Work out the finished part from the listing and answer in its coordinate system (mm). Face numbers are marked on the shaded views. A direction names the side the tool comes from. Give positions to 0.01 mm unless a question says otherwise; leave off trailing zeros. Write each loop counter-clockwise with the first axis right and the second up, starting at its lowest first coordinate (ties: lowest second). Pieces come first, ordered by that corner, then holes.
1) Find section D-D (z = -12.5). Determine the outline of the cut face in (x, y) (3 decimals).
2) Determine the mould class of the marked faces 1, 2 and 3 for opening direction Y: pulls with the +Y half, pulls with the -Y half, needs draft (parallel to the pull), parting line crosses it, or undercut.
3) Find section A-A (y = -3). Determine the outline of the cut face in (x, z).
4) Straight lines are drawn through the part: probe 1 along Z at (x, y) = (-17.5, 8.5); probe 2 along Z at (x, y) = (19.5, 18); probe 3 along X at (y, z) = (-2, -2.5). For each, find the intervals that lie inside material, in ascending order.
5) Find section C-C (z = -2.5). Determine the outline of the cut face in (x, y) (3 decimals).
6) Find section B-B (z = 12.5). Determine the outline of the cut face in (x, y), plus the area to 3 significant figures.
7) Given pin 1 Ø3 at (x, y) = (8.5, 9) entering from -Z; pin 2 Ø8 at (x, y) = (18, 2.5) entering from +Z; pin 3 Ø6.5 at (x, y) = (4, 8.5) entering from -Z, each flat-ended and moving along its own axis, determine where each tip first touches the part or whether it passes through.
8) A tool of negligible diameter and unlimited length cuts with its end or side. For the marked faces 4, 5, 6 and 7, from which of +Z, -Z, +X, -X, +Y, -Y can it reach the whole face along a straight path? Write none if from no direction.
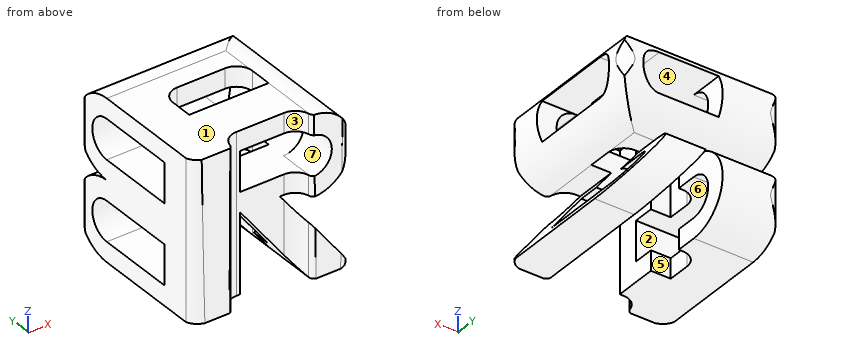
```python
from build123d import *

# Parameters (mm, degrees)
F2_DEPTH = 25
F3_DEPTH = 25
F5_DEPTH = 50


with BuildPart() as f2:
    # F0 (on Front) → F2 (new body, symmetric)
    with BuildSketch(Plane.XZ):
        with BuildLine():
            Line((-25, 25), (-25, -25))
            Line((-25, -25), (-6.25, -25))
            Line((-6.25, -25), (-6.25, 0))
            Line((-6.25, 0), (12.5, -25))
            Line((12.5, -25), (25, -25))
            Line((25, -25), (6.25, 0))
            Line((6.25, 0), (12.5, 0))
            ThreePointArc((12.5, 0), (25, 12.5), (12.5, 25))
            Line((12.5, 25), (-25, 25))
        make_face()
        with BuildLine():
            Line((12.5, 6.25), (-6.25, 6.25))
            Line((-6.25, 6.25), (-6.25, 18.75))
            Line((-6.25, 18.75), (12.5, 18.75))
            ThreePointArc((12.5, 18.75), (18.75, 12.5), (12.5, 6.25))
        make_face(mode=Mode.SUBTRACT)
    extrude(amount=F2_DEPTH, both=True)

    # F1 (on Right) → F3 (intersect, symmetric)
    with BuildSketch(Plane.YZ):
        with BuildLine():
            Line((-25, -25), (12.5, -25))
            ThreePointArc((12.5, -25), (25, -12.5), (12.5, 0))
            ThreePointArc((12.5, 0), (25, 12.5), (12.5, 25))
            Line((12.5, 25), (-24.736971, 25.042934))
            Line((-24.736971, 25.042934), (-25, -25))
        make_face()
        with BuildLine():
            Line((-12.5, -6.25), (12.5, -6.25))
            ThreePointArc((12.5, -6.25), (18.75, -12.5), (12.5, -18.75))
            Line((12.5, -18.75), (-12.5, -18.75))
            Line((-12.5, -18.75), (-12.5, -6.25))
        make_face(mode=Mode.SUBTRACT)
        with BuildLine():
            Line((-12.5, 18.75), (12.5, 18.75))
            ThreePointArc((12.5, 18.75), (18.75, 12.5), (12.5, 6.25))
            Line((12.5, 6.25), (-12.5, 6.25))
            Line((-12.5, 6.25), (-12.5, 18.75))
        make_face(mode=Mode.SUBTRACT)
    extrude(amount=F3_DEPTH, both=True, mode=Mode.INTERSECT)

    # F4 (on face) → F5 (intersect)
    with BuildSketch(Plane.XY.offset(25)):
        with BuildLine():
            ThreePointArc((25.267377, 20.127007), (23.802911, 23.662541), (20.267377, 25.127007))
            Line((20.267377, 25.127007), (-20.267377, 25.127007))
            ThreePointArc((-20.267377, 25.127007), (-23.802911, 23.662541), (-25.267377, 20.127007))
            Line((-25.267377, 20.127007), (-25.267377, -20.127007))
            ThreePointArc((-25.267377, -20.127007), (-23.802911, -23.662541), (-20.267377, -25.127007))
            Line((-20.267377, -25.127007), (-14.361611, -25.127007))
            ThreePointArc((-14.361611, -25.127007), (-13.09501, -24.674819), (-12.401151, -23.522729))
            ThreePointArc((-12.401151, -23.522729), (-10.666503, -20.642503), (-7.5, -19.512033))
            Line((-7.5, -19.512033), (7.5, -19.512033))
            ThreePointArc((7.5, -19.512033), (10.666503, -20.642503), (12.401151, -23.522729))
            ThreePointArc((12.401151, -23.522729), (13.09501, -24.674819), (14.361611, -25.127007))
            Line((14.361611, -25.127007), (20.267377, -25.127007))
            ThreePointArc((20.267377, -25.127007), (23.802911, -23.662541), (25.267377, -20.127007))
            Line((25.267377, -20.127007), (25.267377, 20.127007))
        make_face()
        with BuildLine():
            Line((-7.5, 6.036096), (7.5, 6.036096))
            ThreePointArc((7.5, 6.036096), (11.035534, 4.57163), (12.5, 1.036096))
            Line((12.5, 1.036096), (12.5, -6.036096))
            Line((12.5, -6.036096), (-12.5, -6.036096))
            Line((-12.5, -6.036096), (-12.5, 1.036096))
            ThreePointArc((-12.5, 1.036096), (-11.035534, 4.57163), (-7.5, 6.036096))
        make_face(mode=Mode.SUBTRACT)
    extrude(amount=-F5_DEPTH, mode=Mode.INTERSECT)


solid = f2.part
```
Results:
1. outline: (-25, -21.74) arc R5 ccw to (-21.642, -24.934) - (-13.505, -24.934) arc R2 ccw to (-12.401, -23.523) arc R5 cw to (-7.5, -19.512) - (-6.25, -19.512) - (-6.25, -12.5) - (-25, -12.5) - close; (-25, 18.75) - (-6.25, 18.75) - (-6.25, 25) - (-21.387, 25) arc R5 ccw to (-25, 21.74) - close; (3.125, -19.512) - (7.5, -19.512) arc R5 cw to (12.401, -23.523) arc R2 ccw to (13.505, -24.934) - (15.625, -24.934) - (15.625, -12.5) - (3.125, -12.5) - close; (3.125, 18.75) - (15.625, 18.75) - (15.625, 25) - (3.125, 25) - close
2. face 1: needs draft
2. face 2: undercut
2. face 3: pulls with the -Y half
3. outline: (-25, -25) - (-12.5, -25) - (-12.5, -18.75) - (-25, -18.75) - close; (-25, -6.25) - (-12.5, -6.25) - (-12.5, 6.25) - (-25, 6.25) - close; (-25, 18.75) - (-12.5, 18.75) - (-12.5, 25) - (-25, 25) - close; (12.5, -25) - (25, -25) - (20.31, -18.75) - (12.5, -18.75) - close; (12.5, 0) arc R12.5 ccw to (23.33, 6.25) - (12.5, 6.25) - close; (12.5, 18.75) - (23.33, 18.75) arc R12.5 ccw to (12.5, 25) - close
4. probe 1: z = -25 to -18.75, -6.25 to 6.25, 18.75 to 25
4. probe 2: z = -23.72 to -17.67, 2.14 to 9.53, 15.47 to 22.86
4. probe 3: x = -25 to -12.5
5. outline: (-25, -21.74) arc R5 ccw to (-21.814, -24.882) - (-13.402, -24.882) arc R2 ccw to (-12.401, -23.523) arc R5 cw to (-7.5, -19.512) - (-6.25, -19.512) - (-6.25, -6.036) - (-12.5, -6.036) - (-12.5, 1.036) arc R5 cw to (-7.5, 6.036) - (-6.25, 6.036) - (-6.25, 20) - (-25, 20) - close; (-4.375, -19.512) - (7.5, -19.512) arc R5 cw to (8.125, -19.551) - (8.125, -6.036) - (-4.375, -6.036) - close; (-4.375, 6.036) - (7.5, 6.036) arc R5 cw to (8.125, 5.997) - (8.125, 20) - (-4.375, 20) - close
6. outline: (-25, -21.74) arc R5 ccw to (-22.04, -24.8) - (-13.27, -24.8) arc R2 ccw to (-12.4, -23.52) arc R5 cw to (-7.5, -19.51) - (-6.25, -19.51) - (-6.25, -12.5) - (-25, -12.5) - close; (-25, 18.75) - (-6.25, 18.75) - (-6.25, 25) - (-21.39, 25) arc R5 ccw to (-25, 21.74) - close; (18.75, -24.8) - (22.04, -24.8) arc R5 ccw to (25, -21.74) - (25, -12.5) - (18.75, -12.5) - close; (18.75, 18.75) - (25, 18.75) - (25, 21.74) arc R5 ccw to (21.39, 25) - (18.75, 25) - close
6. area: 422 mm2
7. pin 1: stops at z = -21.67
7. pin 2: stops at z = 24.91
7. pin 3: stops at z = -6.25
8. face 4: none
8. face 5: +Z, -Z
8. face 6: +X, -X
8. face 7: +Y, -Y
